from build123d import *

# Parameters (mm, degrees)
SKETCH_1_W                       = 51.5
SKETCH_1_H                       = 26
SM_BASE_FLANGE_1_DEPTH           = 2
SM_EDGE_FLANGE_1_STRIP_W         = 9.4732
SM_EDGE_FLANGE_1_STRIP_H         = 2
SM_EDGE_FLANGE_1_STRIP_CUT_DEPTH = 26
SM_EDGE_FLANGE_1_DEPTH           = 26
SM_EDGE_FLANGE_2_STRIP_W         = 9.4732
SM_EDGE_FLANGE_2_STRIP_H         = 2
SM_EDGE_FLANGE_2_STRIP_CUT_DEPTH = 26
SM_EDGE_FLANGE_2_DEPTH           = 26
CUT_EXTRUDE_3_DEPTH              = 100
SKETCH_21_R                      = 1
SKETCH_21_R_2                    = 1.5
SKETCH_21_R_3                    = 4
CUT_EXTRUDE_5_DEPTH              = 100
SKETCH_22_R                      = 1.5
SKETCH_22_R_2                    = 6
CUT_EXTRUDE_6_DEPTH              = 3
SKETCH_23_R                      = 1.5
CUT_EXTRUDE_7_DEPTH              = 60


# Sheet-metal steps are written as plain solids
with BuildPart() as part:
    # Sketch 1 → 基体-法兰1 (new body)
    with BuildSketch(Plane.XY):
        with Locations((4.131805158, 0.27256447)):
            Rectangle(SKETCH_1_W, SKETCH_1_H)
    extrude(amount=-SM_BASE_FLANGE_1_DEPTH)

    # 边线-法兰1 strip (across the edge) → 边线-法兰1 strip cut (cut)
    with BuildSketch(Plane(origin=(29.881805158, -12.72743553, 0), x_dir=(-1, 0, 0), z_dir=(0, 1, 0))):
        with Locations((-4, -1)):
            Rectangle(SM_EDGE_FLANGE_1_STRIP_W, SM_EDGE_FLANGE_1_STRIP_H)
    extrude(amount=SM_EDGE_FLANGE_1_STRIP_CUT_DEPTH, mode=Mode.SUBTRACT)

    # 边线-法兰1 section (across the edge) → 边线-法兰1 (add)
    with BuildSketch(Plane(origin=(29.881805158, -12.72743553, 0), x_dir=(-1, 0, 0), z_dir=(0, 1, 0))):
        with BuildLine():
            Line((-2, 0.7366), (-2, 43))
            Line((-2, 43), (0, 43))
            Line((0, 43), (0, 0.7366))
            ThreePointArc((0, 0.7366), (0.215745145, 0.215745145), (0.7366, 0))
            Line((0.7366, 0), (0.7366, -2))
            ThreePointArc((0.7366, -2), (-1.198468417, -1.198468417), (-2, 0.7366))
        make_face()
    extrude(amount=SM_EDGE_FLANGE_1_DEPTH)

    # 边线-法兰2 strip (across the edge) → 边线-法兰2 strip cut (cut)
    with BuildSketch(Plane(origin=(-21.618194842, 13.27256447, 0), x_dir=(1, 0, 0), z_dir=(0, -1, 0))):
        with Locations((-4, -1)):
            Rectangle(SM_EDGE_FLANGE_2_STRIP_W, SM_EDGE_FLANGE_2_STRIP_H)
    extrude(amount=SM_EDGE_FLANGE_2_STRIP_CUT_DEPTH, mode=Mode.SUBTRACT)

    # 边线-法兰2 section (across the edge) → 边线-法兰2 (add)
    with BuildSketch(Plane(origin=(-21.618194842, 13.27256447, 0), x_dir=(1, 0, 0), z_dir=(0, -1, 0))):
        with BuildLine():
            Line((-2, 0.7366), (-2, 43))
            Line((-2, 43), (0, 43))
            Line((0, 43), (0, 0.7366))
            ThreePointArc((0, 0.7366), (0.215745145, 0.215745145), (0.7366, 0))
            Line((0.7366, 0), (0.7366, -2))
            ThreePointArc((0.7366, -2), (-1.198468417, -1.198468417), (-2, 0.7366))
        make_face()
    extrude(amount=SM_EDGE_FLANGE_2_DEPTH)

    # 草图14 → 切除-拉伸3 (cut)
    with BuildSketch(Plane(origin=(31.881805158, 0, 0), x_dir=(0, 0, -1), z_dir=(1, 0, 0))):
        with BuildLine():
            ThreePointArc((-43, 0.27256447), (-39.192388155, 9.464952625), (-30, 13.27256447))
            Line((-30, 13.27256447), (-43, 13.27256447))
            Line((-43, 13.27256447), (-43, 0.27256447))
        make_face()
        with BuildLine():
            Line((-43, -12.72743553), (-30, -12.72743553))
            ThreePointArc((-30, -12.72743553), (-39.192388155, -8.919823686), (-43, 0.27256447))
            Line((-43, 0.27256447), (-43, -12.72743553))
        make_face()
    extrude(amount=-CUT_EXTRUDE_3_DEPTH, mode=Mode.SUBTRACT)

    # 草图21 → 切除-拉伸5 (cut)
    with BuildSketch(Plane(origin=(31.881805158, 0, 0), x_dir=(0, 0, -1), z_dir=(1, 0, 0))):
        with Locations((-25.050252532, 5.222311938)):
            Circle(SKETCH_21_R)
        with Locations((-23, 0.27256447)):
            Circle(SKETCH_21_R_2)
        with Locations((-25.050252532, -4.677182998)):
            Circle(SKETCH_21_R)
        with Locations((-30, -6.72743553)):
            Circle(SKETCH_21_R_2)
        with Locations((-34.949747468, -4.677182998)):
            Circle(SKETCH_21_R)
        with Locations((-37, 0.27256447)):
            Circle(SKETCH_21_R_2)
        with Locations((-34.949747468, 5.222311938)):
            Circle(SKETCH_21_R)
        with Locations((-30, 7.27256447)):
            Circle(SKETCH_21_R_2)
        with Locations((-30, 0.27256447)):
            Circle(SKETCH_21_R_3)
    extrude(amount=-CUT_EXTRUDE_5_DEPTH, mode=Mode.SUBTRACT)

    # 草图22 → 切除-拉伸6 (cut)
    with BuildSketch(Plane.XY):
        with Locations((10.849319579, 6.990078891)):
            Circle(SKETCH_22_R)
        with Locations((10.849319579, -6.444949951)):
            Circle(SKETCH_22_R)
        with Locations((-2.585709264, -6.444949951)):
            Circle(SKETCH_22_R)
        with Locations((-2.585709264, 6.990078891)):
            Circle(SKETCH_22_R)
        with Locations((4.131805158, 0.27256447)):
            Circle(SKETCH_22_R_2)
    extrude(amount=-CUT_EXTRUDE_6_DEPTH, mode=Mode.SUBTRACT)

    # 草图23 → 切除-拉伸7 (cut)
    with BuildSketch(Plane(origin=(31.881805158, 0, 0), x_dir=(0, 0, -1), z_dir=(1, 0, 0))):
        with Locations((-6.7366, 0.27256447)):
            Circle(SKETCH_23_R)
    extrude(amount=-CUT_EXTRUDE_7_DEPTH, mode=Mode.SUBTRACT)


solid = part.part
Design review of the part built by this model. Coordinates are the model's own, in mm. A direction names the side the tool comes from. Coordinates: 2 decimals unless noted, no trailing zeros. Order: outer loops, then holes, each group sorted by start corner. A loop starts at its lowest first (then second) coordinate and runs counter-clockwise, first axis right, second up. Notation, with made-up numbers: (25.5, 86.5) -> (66.5, 86.5) arc R13 cw to (66.5, 107.5) -> close; hole circle Ø11 at (-5.75, -20). An arc over 180 degrees is marked (long way). Use one line per item in the form item = value. Start each with the question number.
(1) For probe 1 along Y at (x, z) = (30.85, 30); probe 2 along X at (y, z) = (0.5, 25.5); probe 3 along Z at (x, y) = (25, -3), list the stretches that pass through material, from the lowest coordinate up.
(2) Insertion check: pin 1 (12 mm diameter, centred on x = 22.5, z = 18.5, fed in from -Y); pin 2 (8 mm diameter, centred on x = 13.5, y = 1, fed in from +Z). Each pin has a flat end and moves straight along its axis. Give the tip position at first contact, or say it passes through.
(3) Add section D-D on y = 3.25. State the section outline as (x, z) points.
(4) The part is to be moulded in two halves that separate along Y. For faces 3 (the cylindrical face through (30.9, 0.3, 24.5)), 4 (the flat face through (31.882, 0, 17)), 5 (the flat face through (4, -12.727, -1)), 6 (the flat face through (4.26, 13.273, -0.15)), say which applies: +Y half, -Y half, draft (parallel to the pull), parting line (faces both ways), or undercut.
(5) Add section C-C on x = 1.5. State the section outline as (y, z) points, plus the area to 3 significant figures.
(6) Add section B-B on x = 11. State the section outline as (y, z) points, plus the area to 3 significant figures.
(7) Add section A-A on z = 23. State the section outline as (x, y) points.
(8) For faces 1 (the cylindrical face through (30.9, 4.24, 30.52)), 2 (the flat face through (-21.618, 0, 17)), list the 3-axis set-ups (+Z, -Z, +X, -X, +Y, -Y) from which the entire face can be reached by the end or side of a thin tool; tool diameter is ignored.
Answer block:
q1.probe_1 = -12.73 to -8.23, -5.23 to -3.73, 4.27 to 5.77, 8.77 to 13.27
q1.probe_2 = -23.62 to -21.62, 29.88 to 31.88
q1.probe_3 = -2 to 0
q2.pin_1 = through
q2.pin_2 = 0
q3.outline = (-23.62, 0.74) arc R2.74 ccw to (-20.88, -2) -> (-1.08, -2) -> (-1.08, 0) -> (-20.88, 0) arc R0.74 cw to (-21.62, 0.74) -> (-21.62, 27.33) -> (-23.62, 27.33) -> close; (-23.62, 32.67) -> (-21.62, 32.67) -> (-21.62, 42.65) -> (-23.62, 42.65) -> close; (9.34, -2) -> (29.15, -2) arc R2.74 ccw to (31.88, 0.74) -> (31.88, 27.33) -> (29.88, 27.33) -> (29.88, 0.74) arc R0.74 cw to (29.15, 0) -> (9.34, 0) -> close; (29.88, 32.67) -> (31.88, 32.67) -> (31.88, 42.65) -> (29.88, 42.65) -> close
q4.face_3 = undercut
q4.face_4 = draft
q4.face_5 = -Y half
q4.face_6 = +Y half
q5.outline = (-12.73, -2) -> (-5.12, -2) -> (-5.12, 0) -> (-12.73, 0) -> close; (5.66, -2) -> (13.27, -2) -> (13.27, 0) -> (5.66, 0) -> close
q5.area = 30.4 mm²
q6.outline = (-12.73, -2) -> (-7.94, -2) -> (-7.94, 0) -> (-12.73, 0) -> close; (-4.95, -2) -> (5.5, -2) -> (5.5, 0) -> (-4.95, 0) -> close; (8.48, -2) -> (13.27, -2) -> (13.27, 0) -> (8.48, 0) -> close
q6.area = 40.1 mm²
q7.outline = (-23.62, -12.73) -> (-21.62, -12.73) -> (-21.62, -1.23) -> (-23.62, -1.23) -> close; (-23.62, 1.77) -> (-21.62, 1.77) -> (-21.62, 13.27) -> (-23.62, 13.27) -> close; (29.88, -12.73) -> (31.88, -12.73) -> (31.88, -1.23) -> (29.88, -1.23) -> close; (29.88, 1.77) -> (31.88, 1.77) -> (31.88, 13.27) -> (29.88, 13.27) -> close
q8.face_1 = +X, -X
q8.face_2 = +Z, +Y, -Y
